Source: CAD feature listing. Evaluate the final solid. Frame: model axes, mm. A direction names the side the tool comes from. Coordinates: 2 decimals unless noted, no trailing zeros. Order: outer loops, then holes, each group sorted by start corner. A loop starts at its lowest first (then second) coordinate and runs counter-clockwise, first axis right, second up.
```python
from build123d import *

# Parameters (mm, degrees)
BOSS_EXTRUDE1_DEPTH          = 0.4445
F_97_0_0059_DIAMETER_HOLE1_D = 2.921
SKETCH7_W                    = 0.500000016
SKETCH7_H                    = 0.889
BOSS_EXTRUDE2_DEPTH          = 6.35
SKETCH11_W                   = 6.35
SKETCH11_H                   = 0.889
BOSS_EXTRUDE3_DEPTH          = 0.127
SKETCH12_W                   = 6.35
SKETCH12_H                   = 0.889
BOSS_EXTRUDE4_DEPTH          = 0.127


with BuildPart() as part:
    # Sketch1 → Boss-Extrude1 (new, symmetric)
    with BuildSketch(Plane(origin=(0, 0, 0), x_dir=(1, 0, 0), z_dir=(0, 1, 0))):
        Polygon((-41.424046485, -10.283259465), (-41.424046485, -12.505759465), (-47.774046485, -12.505759465), (-47.774046485, -6.155759465), (-41.424046485, -6.155759465), (-41.424046485, -8.378259465), (-9.674046485, -8.378259465), (-9.674046485, -6.155759465), (-3.324046485, -6.155759465), (-3.324046485, -12.505759465), (-9.674046485, -12.505759465), (-9.674046485, -10.283259465), align=None)
    extrude(amount=BOSS_EXTRUDE1_DEPTH, both=True)

    # #97 (0.0059) Diameter Hole1 (through all)
    with Locations(Plane(origin=(0, 0.4445, 0), x_dir=(-1, 0, 0), z_dir=(0, 1, 0))):
        with Locations((44.599046485, 9.330759465)):
            f_97_0_0059_diameter_hole1 = Hole(F_97_0_0059_DIAMETER_HOLE1_D / 2)

    # Mirror1: #97 (0.0059) Diameter Hole1 across plane
    add(f_97_0_0059_diameter_hole1.mirror(Plane(origin=(-25.549046485, 0, 0), x_dir=(0, 0, 1), z_dir=(1, 0, 0))), mode=Mode.SUBTRACT)

    # Sketch7 → Boss-Extrude2 (add)
    with BuildSketch(Plane.XY.offset(10.283259465)):
        with Locations((-25.549046485, 0)):
            Rectangle(SKETCH7_W, SKETCH7_H)
    extrude(amount=BOSS_EXTRUDE2_DEPTH)

    # Sketch11 → Boss-Extrude3 (add)
    with BuildSketch(Plane.ZY.offset(25.799046493)):
        with Locations((13.458259465, 0)):
            Rectangle(SKETCH11_W, SKETCH11_H)
    extrude(amount=BOSS_EXTRUDE3_DEPTH)

    # Sketch12 → Boss-Extrude4 (add)
    with BuildSketch(Plane(origin=(-25.299046477, 0, 0), x_dir=(0, 0, -1), z_dir=(1, 0, 0))):
        with Locations((-13.458259465, 0)):
            Rectangle(SKETCH12_W, SKETCH12_H)
    extrude(amount=BOSS_EXTRUDE4_DEPTH)


solid = part.part
```
1. Section query A-A, the plane x = -7.5. Output: boundary loops of the cut face in (y, z).
2. Section query C-C, the plane x = -22.5. Output: boundary loops of the cut face in (y, z), plus the area to 3 significant figures.
3. Draft query along Z for faces 1 (the flat face through (-41.424, 0, 7)), 2 (the cylindrical face through (-45.675, -0.006, 10.318)), 3 (the flat face through (-26, 0, 8.378)), 4 (the cylindrical face through (-5.423, -0.006, 10.318)). Return one class per face: +Z half, -Z half, draft (parallel to the pull), parting line (faces both ways), or undercut.
4. Access query for faces 5 (the flat face through (-9.674, 0, 7)), 6 (the flat face through (-45, 0, 12.506)), 7 (the flat face through (-6, 0, 12.506)), 8 (the flat face through (-7, 0, 6.156)), 9 (the flat face through (-41.424, 0, 11)). Directions: +Z, -Z, +X, -X, +Y, -Y. A direction counts if a zero-diameter tool reaches every point of the face in a straight line with its end or side. Return the directions, or none.
5. Section query B-B, the plane y = -0.25. Output: boundary loops of the cut face in (x, z).
6. Material intervals for line 1 along X through (y, z) = (-0.2, 11); line 2 along X through (y, z) = (-0.2, 7.75); line 3 along Z through (x, y) = (-44.5, 0.3), sorted ascending.
7. Contact query for a flat-ended pin moving along its axis: P1, Ø5, axis at x = -17.5, z = 10.5, coming from the -Y side. Output: stop coordinate, or through.
Answer key:
1. outline: (-0.44, 6.16) - (0.44, 6.16) - (0.44, 8.27) - (-0.44, 8.27) - close; (-0.44, 10.39) - (0.44, 10.39) - (0.44, 12.51) - (-0.44, 12.51) - close
2. outline: (-0.44, 8.38) - (0.44, 8.38) - (0.44, 10.28) - (-0.44, 10.28) - close
2. area: 1.69 mm2
3. face 1: draft
3. face 2: undercut
3. face 3: -Z half
3. face 4: undercut
4. face 5: -Z, +Y, -Y
4. face 6: +Z, -X, +Y, -Y
4. face 7: +Z, +X, +Y, -Y
4. face 8: -Z, +X, -X, +Y, -Y
4. face 9: +Z, +Y, -Y
5. outline: (-47.77, 6.16) - (-41.42, 6.16) - (-41.42, 8.38) - (-9.67, 8.38) - (-9.67, 6.16) - (-3.32, 6.16) - (-3.32, 12.51) - (-9.67, 12.51) - (-9.67, 10.28) - (-25.17, 10.28) - (-25.17, 16.63) - (-25.93, 16.63) - (-25.93, 10.28) - (-41.42, 10.28) - (-41.42, 12.51) - (-47.77, 12.51) - close; hole circle Ø2.92 at (-44.6, 9.33); hole circle Ø2.92 at (-6.5, 9.33)
6. line 1: x = -47.77 to -41.42, -25.93 to -25.17, -9.67 to -3.32
6. line 2: x = -47.77 to -41.42, -9.67 to -3.32
6. line 3: z = 6.16 to 7.87, 10.79 to 12.51
7. P1: stops at y = -0.44
